The figure shows three views and two pictorial views of one solid part (mm, origin at its lowest corner). Answer the questions. A direction names the side the tool comes from. Give positions to 0.01 mm unless a question says otherwise; leave off trailing zeros. Write each loop counter-clockwise with the first axis right and the second up, starting at its lowest first coordinate (ties: lowest second). Pieces come first, ordered by that corner, then holes. Notation, with made-up numbers: M 52,-7.75 L 87,-7.75 A21 cw 87,12.25 Z; hole C -29.5,40 d11. An arc over 180 degrees is marked long. Return JSON: item names as keys, results as strings.
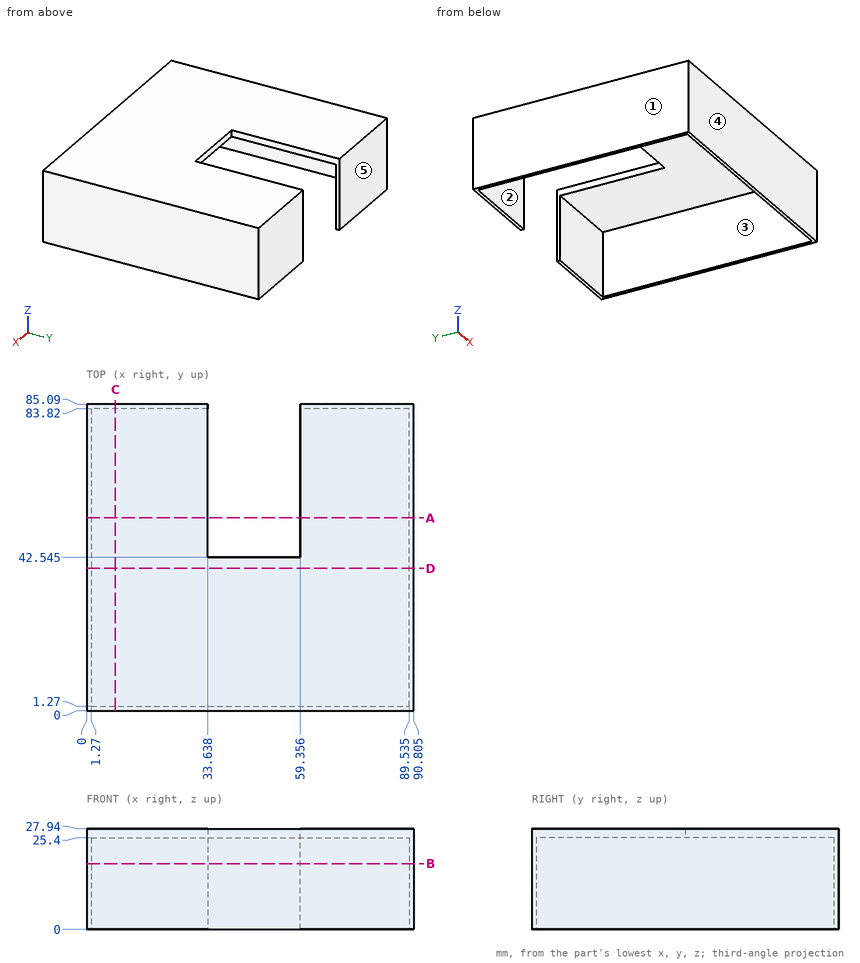
Item 1: Find the intervals of material crossed by line 1 (X direction, y = 69.5, z = 17.5) (1 decimal); line 2 (Y direction, x = 66.5, z = 4); line 3 (X direction, y = 52, z = 26.75) (1 decimal), in increasing order.
Geometry results:
{"line 1": "x = 0 to 1.3, 89.5 to 90.8", "line 2": "y = 0 to 1.27, 83.82 to 85.09", "line 3": "x = 0 to 33.6, 59.4 to 90.8"}
Item 2: Determine the mould class of the marked faces 3, 4 and 5 for opening direction Y: +Y half, -Y half, draft (parallel to the pull), parting line (faces both ways), or undercut.
Geometry results:
{"face 3": "undercut", "face 4": "-Y half", "face 5": "+Y half"}
Item 3: Given pin 1 Ø7.5 at (x, z) = (43.5, 11) entering from +Y; pin 2 Ø3 at (x, z) = (48.5, 26) entering from +Y (3 decimals); pin 3 Ø12 at (x, y) = (18, 13) entering from -Z, each flat-ended and moving along its own axis, determine where each tip first touches the part or whether it passes through.
Geometry results:
{"pin 1": "stops at y = 1.27", "pin 2": "stops at y = 42.545", "pin 3": "stops at z = 25.4"}
Item 4: Which of the six approach directions +Z, -Z, +X, -X, +Y, -Y give full straight-line access (tool end or side, diameter ignored) to the marked faces 1 and 2?
Geometry results:
{"face 1": "+Z, -Z, -X, +Y, -Y", "face 2": "-Z"}
Item 5: A cutting plane is placed at D-D, the plane y = 39.5. Write down the section's boundary in (x, z) (1 decimal), plus the area to 3 significant figures.
Geometry results:
{"outline": "M 0,0 L 1.3,0 L 1.3,25.4 L 89.5,25.4 L 89.5,0 L 90.8,0 L 90.8,27.9 L 0,27.9 Z", "area": "295 mm2"}
Item 6: A cutting plane is placed at B-B, the plane z = 18.25. Write down the section's boundary in (x, y) (1 decimal).
Geometry results:
{"outline": "M 0,0 L 90.8,0 L 90.8,85.1 L 59.4,85.1 L 59.4,83.8 L 89.5,83.8 L 89.5,1.3 L 1.3,1.3 L 1.3,83.8 L 33.6,83.8 L 33.6,85.1 L 0,85.1 Z"}
Item 7: A cutting plane is placed at A-A, the plane y = 53.5. Write down the section's boundary in (x, z) (1 decimal).
Geometry results:
{"outline": "M 0,0 L 1.3,0 L 1.3,25.4 L 33.6,25.4 L 33.6,27.9 L 0,27.9 Z; M 59.4,25.4 L 89.5,25.4 L 89.5,0 L 90.8,0 L 90.8,27.9 L 59.4,27.9 Z"}
Item 8: A cutting plane is placed at C-C, the plane x = 8. Write down the section's boundary in (y, z).
Geometry results:
{"outline": "M 0,0 L 1.27,0 L 1.27,25.4 L 83.82,25.4 L 83.82,0 L 85.09,0 L 85.09,27.94 L 0,27.94 Z"}
